from build123d import *

# Parameters (mm, degrees)
F0_W     = 28
F0_H     = 34
F0_R     = 11.15
F1_DEPTH = 15
F0_R_2   = 6
F2_DEPTH = 2
F3_R     = 1.65
F4_DEPTH = 6
F3_R_2   = 2.8
F5_DEPTH = 2.5
F7_R     = 5
F8_R     = 2


with BuildPart() as f1:
    # F0 (on Top) → F1 (new body)
    with BuildSketch(Plane.XY):
        Rectangle(F0_W, F0_H)
        with Locations((0, 0.35)):
            Circle(F0_R, mode=Mode.SUBTRACT)
        Polygon((14, -17), (-14, -17), (-25.5, -17), (-25.5, -23), (25.5, -23), (25.5, -17), align=None)
    extrude(amount=F1_DEPTH)

    # F0 (on Top) → F2 (join)
    with BuildSketch(Plane.XY):
        with Locations((0, 0.35)):
            Circle(F0_R)
        with Locations((0, 0.35)):
            Circle(F0_R_2, mode=Mode.SUBTRACT)
    extrude(amount=F2_DEPTH)

    # F3 (on face) → F4 (cut, through all)
    with BuildSketch(Plane(origin=(0, -17, 0), x_dir=(-1, 0, 0), z_dir=(0, 1, 0))):
        with Locations((19.75, 7.5)):
            Circle(F3_R)
    extrude(amount=-F4_DEPTH, mode=Mode.SUBTRACT)

    # F3 (on face) → F5 (cut)
    with BuildSketch(Plane(origin=(0, -17, 0), x_dir=(-1, 0, 0), z_dir=(0, 1, 0))):
        with Locations((19.75, 7.5)):
            Circle(F3_R_2)
        with Locations((19.75, 7.5)):
            Circle(F3_R, mode=Mode.SUBTRACT)
    extrude(amount=-F5_DEPTH, mode=Mode.SUBTRACT)

    # F6: F1 across plane


with BuildPart() as f1_1:
    add(f1.part)
    add(f1.part.mirror(Plane.YZ), mode=Mode.INTERSECT)

    # F7
    f7_edges = [f1_1.edges().sort_by_distance(p)[0] for p in [
        (-14, 17, 7.5),
        (14, 17, 7.5),
    ]]
    fillet(f7_edges, radius=F7_R)

    # F8
    f8_edges = [f1_1.edges().sort_by_distance(p)[0] for p in [
        (-11.15, 0.35, 15),
    ]]
    fillet(f8_edges, radius=F8_R)


solid = f1_1.part
Geometry: final body of the model. Coordinates: model frame, mm. A direction names the side the tool comes from. Give positions to 0.01 mm unless a question says otherwise; leave off trailing zeros. Loops run counter-clockwise (first coordinate to the right, second up) from the corner with the lowest first, then second, coordinate; pieces in that order, holes last. Notation, with made-up numbers: M 55,55 L 74,55 A28 ccw 74,79 Z; hole C 4.5,-1.5 d1. An arc over 180 degrees is marked long. Put each result on its own line as item: value.
1) First-contact query: P1, Ø6, axis at x = 18.5, z = 8, coming from the +Y side; P2, Ø4.5, axis at x = -19.75, z = 7.5, coming from the +Y side; P3, Ø2, axis at y = 2.5, z = 9, coming from the +X side. Flat tips, straight axial feed; report the tip coordinate or a pass-through.
Computed values:
P1: stops at y = -17
P2: stops at y = -19.5
P3: stops at x = 14
2) Material intervals for L1, parallel to Y at x = 0, z = 1.6; L2, parallel to X at y = 0.35, z = 1.55; L3, parallel to Z at x = -19.75, y = -21.2, sorted ascending. Write a range as from..to.
Computed values:
L1: y = -23..-5.65, 6.35..17
L2: x = -14..-6, 6..14
L3: z = 0..5.85, 9.15..15
3) Cut plane C-C, the plane z = 11. Return the cut outline in (x, y), plus the area to 3 significant figures.
Computed values:
outline: M -25.5,-23 L 25.5,-23 L 25.5,-17 L 14,-17 L 14,12 A5 ccw 9,17 L -9,17 A5 ccw -14,12 L -14,-17 L -25.5,-17 Z; hole C 0,0.35 d22.3
area: 857 mm^2
4) Cut plane B-B, the plane x = 0. Return the cut outline in (y, z), plus the area to 3 significant figures.
Computed values:
outline: M -23,0 L -5.65,0 L -5.65,2 L -10.8,2 L -10.8,13 A2 ccw -12.8,15 L -23,15 Z; M 6.35,0 L 17,0 L 17,15 L 13.5,15 A2 ccw 11.5,13 L 11.5,2 L 6.35,2 Z
area: 284 mm^2
5) Cut plane A-A, the plane z = 6.75. Return the cut outline in (x, y).
Computed values:
outline: M -25.5,-23 L -21.22,-23 L -21.22,-19.5 L -22.45,-19.5 L -22.45,-17 L -25.5,-17 Z; M -18.28,-23 L 18.28,-23 L 18.28,-19.5 L 17.05,-19.5 L 17.05,-17 L 14,-17 L 14,12 A5 ccw 9,17 L -9,17 A5 ccw -14,12 L -14,-17 L -17.05,-17 L -17.05,-19.5 L -18.28,-19.5 Z; M 21.22,-23 L 25.5,-23 L 25.5,-17 L 22.45,-17 L 22.45,-19.5 L 21.22,-19.5 Z; hole C 0,0.35 d22.3
6) Mould query, pull axis X, two halves, no side actions, for faces 1 (the cylindrical face through (18.44, -21.23, 6.5)), 2 (the flat face through (0, -23, 7)), 3 (the flat face through (-21, -19.5, 6)), 4 (the cylindrical face through (12, 16, 8)). Classes: released by +X, released by -X, zero draft, split by the parting line, or undercut.
Computed values:
face 1: undercut
face 2: zero draft
face 3: undercut
face 4: released by +X
7) Reachability of faces 5 (the cylindrical face through (5.994, 9.752, 7.423)), 6 (the flat face through (14, -3, 7)), 7 (the flat face through (-14, -3, 7)), 8 (the flat face through (21, -19.5, 6)), 9 (the flat face through (0, 17, 7)) from +Z, -Z, +X, -X, +Y, -Y: full face, straight path, thin tool, end or side. Return the list, or none.
Computed values:
face 5: +Z
face 6: +Z, -Z, +X, +Y
face 7: +Z, -Z, -X, +Y
face 8: +Y
face 9: +Z, -Z, +X, -X, +Y
8) Cut plane D-D, the plane y = 0.35. Return the cut outline in (x, z), plus the area to 3 significant figures.
Computed values:
outline: M -14,0 L -6,0 L -6,2 L -11.15,2 L -11.15,13 A2 ccw -13.15,15 L -14,15 Z; M 6,0 L 14,0 L 14,15 L 13.15,15 A2 ccw 11.15,13 L 11.15,2 L 6,2 Z
area: 104 mm^2
